For this review, take the finished solid that the model builds, in its own axes (mm). A direction names the side the tool comes from. Coordinates: 2 decimals unless noted, no trailing zeros. Order: outer loops, then holes, each group sorted by start corner. A loop starts at its lowest first (then second) coordinate and runs counter-clockwise, first axis right, second up. Notation, with made-up numbers: (8.25, 6.5) - (21.25, 6.5) arc R26 cw to (21.25, 25.5) - close; hole circle Ø4 at (-11, 75.25). An arc over 180 degrees is marked (long way). One line per item, written item: value. Start each with the question number.
(1) Consider section C-C on z = 3. Write out the cut boundary in (x, y).
(2) For faces 1 (the flat face through (9, 5, 8)), 2 (the flat face through (6, 3, 15)), 3 (the flat face through (6, 6, 8)), 4 (the flat face through (35, 3, 37)), 5 (the flat face through (25, 3, 38)), list the 3-axis set-ups (+Z, -Z, +X, -X, +Y, -Y) from which the entire face can be reached by the end or side of a thin tool; tool diameter is ignored.
(3) Consider section A-A on z = 37.5. Write out the cut boundary in (x, y).
(4) Consider section D-D on x = 5.75. Write out the cut boundary in (y, z), then the cut area to 3 significant figures.
(5) To check wall thickness, follow line 1 along X through (y, z) = (1.5, 37.5); line 2 along X through (y, z) = (3.9, 6); line 3 along Y through (x, z) = (5.75, 11). State the ranges of each line that lie inside material, in increasing order.
(6) Mouldability with a two-part tool opening along Z and no side actions: class faces 6 (the cylindrical face through (30.05, 3.04, 36.25)), 7 (the flat face through (30, 6, 36)), 8 (the flat face through (54, 3, 15)), 9 (the flat face through (54, 5, 16)) as released by +Z, released by -Z, zero draft, split by the parting line, or undercut.
(7) Clearance check with flat-ended pins moving along their axes: pin 1 (0.9 mm diameter, centred on x = 6, y = 4.5, fed in from +Z); pin 2 (1.5 mm diameter, centred on y = 4, z = 25, fed in from -X); pin 3 (2 mm diameter, centred on y = 3, z = 19, fed in from -X) (3 decimals); pin 4 (2.5 mm diameter, centred on x = 54.5, y = 4, fed in from +Z). State where each tip first meets the part, or that it passes through.
```python
from build123d import *

# Parameters (mm, degrees)
ESQUISSE1_W             = 60
ESQUISSE1_H             = 6
BOSS_EXTRU_1_DEPTH      = 60
ESQUISSE2_R             = 1.25
ENL_V_MAT_EXTRU_1_DEPTH = 15
ESQUISSE3_R             = 1.25
ENL_V_MAT_EXTRU_2_DEPTH = 15
ESQUISSE4_W             = 10
ESQUISSE4_H             = 11
ENL_V_MAT_EXTRU_3_DEPTH = 3
ENL_V_MAT_EXTRU_4_DEPTH = 52
CHANFREIN1_SIZE2        = 6.433520762
CHANFREIN1_SIZE         = 3
ESQUISSE6_W             = 2.5
ESQUISSE6_H             = 6
ENL_V_MAT_EXTRU_5_DEPTH = 40


with BuildPart() as part:
    # Esquisse1 → Boss.-Extru.1 (new body)
    with BuildSketch(Plane.XY):
        with Locations((30, 3)):
            Rectangle(ESQUISSE1_W, ESQUISSE1_H)
    extrude(amount=BOSS_EXTRU_1_DEPTH)

    # Esquisse2 → Enlèv. mat.-Extru.1 (cut)
    with BuildSketch(Plane(origin=(0, 0, 0), x_dir=(-1, 0, 0), z_dir=(0, 0, -1))):
        with Locations((-54, 3)):
            Circle(ESQUISSE2_R)
        with Locations((-5.75, 3)):
            Circle(ESQUISSE2_R)
    extrude(amount=-ENL_V_MAT_EXTRU_1_DEPTH, mode=Mode.SUBTRACT)

    # Esquisse3 → Enlèv. mat.-Extru.2 (cut)
    with BuildSketch(Plane(origin=(0, 6, 0), x_dir=(1, 0, 0), z_dir=(0, 1, 0))):
        with Locations(Location((30, -37.5, 0), (0, 0, 270))):
            Circle(ESQUISSE3_R)
    extrude(amount=-ENL_V_MAT_EXTRU_2_DEPTH, mode=Mode.SUBTRACT)

    # Esquisse4 → Enlèv. mat.-Extru.3 (cut)
    with BuildSketch(Plane(origin=(0, 6, 0), x_dir=(1, 0, 0), z_dir=(0, 1, 0))):
        Polygon((0, -16), (9, -16), (9, 0), (51, 0), (51, -16), (60, -16), (60, -60), (0, -60), align=None)
        with Locations((30, -37.5)):
            Rectangle(ESQUISSE4_W, ESQUISSE4_H, mode=Mode.SUBTRACT)
    extrude(amount=-ENL_V_MAT_EXTRU_3_DEPTH, mode=Mode.SUBTRACT)

    # Esquisse5 → Enlèv. mat.-Extru.4 (cut)
    with BuildSketch(Plane(origin=(0, 3, 0), x_dir=(1, 0, 0), z_dir=(0, 1, 0))):
        Polygon((60, -16), (35, -32), (35, -43), (25, -43), (25, -32), (0, -16), (-21.594855386, -85.475485762), (75.414479662, -69.930764824), align=None)
    extrude(amount=-ENL_V_MAT_EXTRU_4_DEPTH, mode=Mode.SUBTRACT)

    # Chanfrein1
    chanfrein1_edges = [part.edges().sort_by_distance(p)[0] for p in [
        (30, 3, 32),
    ]]
    chanfrein1_side = [part.faces().sort_by_distance(p)[0] for p in [
        (30, 3.06, 32),
    ]]
    chamfer(chanfrein1_edges, length=CHANFREIN1_SIZE - 0.0001, length2=CHANFREIN1_SIZE2 - 0.0001, reference=chanfrein1_side[0])  # a hair under: the kernel refuses the full size

    # Esquisse6 → Enlèv. mat.-Extru.5 (cut)
    with BuildSketch(Plane(origin=(0, 0, 0), x_dir=(-1, 0, 0), z_dir=(0, 0, -1))):
        with Locations((-58.75, 3)):
            Rectangle(ESQUISSE6_W, ESQUISSE6_H)
        with Locations((-1.25, 3)):
            Rectangle(ESQUISSE6_W, ESQUISSE6_H)
    extrude(amount=-ENL_V_MAT_EXTRU_5_DEPTH, mode=Mode.SUBTRACT)


solid = part.part
```
Geometry check:
1. outline: (2.5, 0) - (57.5, 0) - (57.5, 6) - (51, 6) - (51, 3) - (9, 3) - (9, 6) - (2.5, 6) - close; hole circle Ø2.5 at (5.75, 3); hole circle Ø2.5 at (54, 3)
2. face 1: +Z, -Z, +Y
2. face 2: -Z
2. face 3: +Z, -Z, +X, -X, +Y
2. face 4: +Z, +X, +Y, -Y
2. face 5: +Z, -X, +Y, -Y
3. outline: (25, 0) - (28.75, 0) - (28.75, 6) - (25, 6) - close; (31.25, 0) - (35, 0) - (35, 6) - (31.25, 6) - close
4. outline: (0, 0) - (1.75, 0) - (1.75, 15) - (4.25, 15) - (4.25, 0) - (6, 0) - (6, 16) - (3, 16) - (3, 19.68) - (0, 19.68) - close
4. area: 69.5 mm^2
5. line 1: x = 25 to 28.75, 31.25 to 35
5. line 2: x = 2.5 to 4.88, 6.62 to 9, 51 to 53.13, 54.87 to 57.5
5. line 3: y = 0 to 1.75, 4.25 to 6
6. face 6: undercut
6. face 7: zero draft
6. face 8: released by -Z
6. face 9: released by +Z
7. pin 1: stops at z = 16
7. pin 2: passes through
7. pin 3: stops at x = 3.125
7. pin 4: stops at z = 20
